Geometry check sheet. Reference: the model listing, model coordinates, mm. A direction names the side the tool comes from. Round coordinates to 2 decimals unless told otherwise and drop trailing zeros. Write each loop counter-clockwise with the first axis right and the second up, starting at its lowest first coordinate (ties: lowest second). Pieces come first, ordered by that corner, then holes. Notation, with made-up numbers: M 45,34.5 L 59,34.5 A17 ccw 59,50.5 Z; hole C 5,79.25 d5. An arc over 180 degrees is marked long. Use a Markdown table: item, result.
```python
from build123d import *

# Parameters (mm, degrees)
F0_W     = 60
F0_H     = 90
F1_DEPTH = 30
F2_R     = 20
F3_W     = 10
F3_H     = 15
F4_DEPTH = 90.001
F7_DEPTH = 40.001


with BuildPart() as f1:
    # F0 (on Top) → F1 (new body)
    with BuildSketch(Plane.XY):
        with Locations((30, 45)):
            Rectangle(F0_W, F0_H)
    extrude(amount=F1_DEPTH)

    # F2
    f2_edges = [f1.edges().sort_by_distance(p)[0] for p in [
        (60, 45, 30),
    ]]
    fillet(f2_edges, radius=F2_R)

    # F3 (on face) → F4 (cut, through all)
    with BuildSketch(Plane.XZ):
        with Locations((30, 22.5)):
            Rectangle(F3_W, F3_H)
    extrude(amount=-F4_DEPTH, mode=Mode.SUBTRACT)

    # F6 (on offset) → F7 (cut, through all)
    with BuildSketch(Plane(origin=(20, 0, 0), x_dir=(0, -1, 0), z_dir=(-1, 0, 0))):
        Polygon((-20, 30), (0, 0), (0, 30), align=None)
    extrude(amount=-F7_DEPTH, mode=Mode.SUBTRACT)


solid = f1.part
```
Item 1: Cross-section at D-D, the plane x = 55. Record the cut outline in (y, z), and give its area (3 significant figures).
Outcome:
| item | result |
|---|---|
| outline | M 0,0 L 90,0 L 90,23.23 L 15.49,23.23 Z |
| area | 1,910 mm2 |
Item 2: Access from +Z, -Z, +X, -X, +Y, -Y to the whole of each face (thin tool, end or side, straight path). Record for faces 1 (the face through (20, 6, 22)), 2 (the face through (10, 0, 15)), 3 (the face through (30, 49, 15)).
Outcome:
| item | result |
|---|---|
| face 1 | +Z, +X, -Y |
| face 2 | +Z, -Z, +X, -X, -Y |
| face 3 | +Z, +Y, -Y |
Item 3: Cross-section at B-B, the plane z = 19. Record the cut outline in (x, y), and give its area (3 significant figures).
Outcome:
| item | result |
|---|---|
| outline | M 0,0 L 20,0 L 20,12.67 L 25,12.67 L 25,90 L 0,90 Z; M 35,12.67 L 57.86,12.67 L 57.86,90 L 35,90 Z |
| area | 3,950 mm2 |
Item 4: Mould release check, pull along X, two halves, no side actions. Record for faces 4 (the face through (12, 46, 30)), 5 (the face through (25, 49, 22)), 6 (the face through (35, 49, 22)), 7 (the face through (0, 44, 15)): +X half, -X half, draft (parallel to the pull), parting line (faces both ways), or undercut.
Outcome:
| item | result |
|---|---|
| face 4 | draft |
| face 5 | undercut |
| face 6 | undercut |
| face 7 | -X half |
Item 5: Material ranges on line 1 along Y through (x, z) = (32.5, 10); line 2 along X through (y, z) = (72, 23); line 3 along X through (y, z) = (11.5, 26), recorded low to high. Write a range as from..to.
Outcome:
| item | result |
|---|---|
| line 1 | y = 6.67..90 |
| line 2 | x = 0..25, 35..55.2 |
| line 3 | x = 0..20 |
Item 6: Go/stop test with flat-tipped pins: pin 1 (12 mm diameter, centred on y = 51, z = 23.5, fed in from -X); pin 2 (3 mm diameter, centred on x = 28.5, y = 48, fed in from +Z); pin 3 (4 mm diameter, centred on y = 47, z = 23.5, fed in from +X); pin 4 (1 mm diameter, centred on x = 48.5, z = 25, fed in from -Y). Record where each tip stops, or that it passes through.
Outcome:
| item | result |
|---|---|
| pin 1 | stops at x = 0 |
| pin 2 | stops at z = 15 |
| pin 3 | stops at x = 56.36 |
| pin 4 | stops at y = 16.33 |
Item 7: Cross-section at A-A, the plane y = 56. Record the cut outline in (x, z).
Outcome:
| item | result |
|---|---|
| outline | M 0,0 L 60,0 L 60,10 A20 ccw 40,30 L 35,30 L 35,15 L 25,15 L 25,30 L 0,30 Z |
Item 8: Cross-section at C-C, the plane z = 7. Record the cut outline in (x, y), and give its area (3 significant figures).
Outcome:
| item | result |
|---|---|
| outline | M 0,0 L 20,0 L 20,4.67 L 60,4.67 L 60,90 L 0,90 Z |
| area | 5,210 mm2 |
